For this review, take the finished solid that the model builds, in its own axes (mm). Face numbers are marked on the shaded views. A direction names the side the tool comes from. Give positions to 0.01 mm unless a question says otherwise; leave off trailing zeros. Order: outer loops, then holes, each group sorted by start corner. A loop starts at its lowest first (then second) coordinate and runs counter-clockwise, first axis right, second up.
Item 1: For P1, Ø10, axis at x = 96.5, z = -7.5, coming from the -Y side; P2, Ø4, axis at x = 93, z = -7, coming from the +Y side; P3, Ø10, axis at x = 60.5, y = -6.5, coming from the +Z side, all flat-tipped, find the tip position at first contact; note any pin that passes through.
Item 2: Consider section C-C (x = 74). Give the boundary of the cut face in (y, z).
Item 3: Machinability: for the marked faces 1 and 2, which of the approach directions +Z, -Z, +X, -X, +Y, -Y give a long, thin tool a straight path to every point of the face, cutting with its end or side? Answer none if there is none.
Item 4: Consider section D-D (x = 37.5). Give the boundary of the cut face in (y, z), plus the area to 3 significant figures.
Item 5: For probe 1 along X at (y, z) = (-46, -6); probe 2 along Y at (x, z) = (112, -20.5); probe 3 along Z at (x, y) = (134.5, -69), list the stretches that pass through material, from the lowest coordinate up.
Item 6: Consider section B-B (z = -21.5). Give the boundary of the cut face in (x, y).
Item 7: Consider section A-A (y = -44.45). Give the boundary of the cut face in (x, z) (3 decimals).
Item 8: The part is to be moulded in two halves that separate along Y. For the marked faces 3, 4, 5 and 6, say which applies: released by +Y, released by -Y, zero draft, split by the parting line, or undercut.
```python
from build123d import *

# Parameters (mm, degrees)
F0_W     = 165.1
F0_H     = 31.75
F1_DEPTH = 88.9
F3_DEPTH = 165.101
F4_W     = 165.1
F4_H     = 12.7
F5_DEPTH = 12.7
F6_W     = 165.1
F6_H     = 12.7
F7_DEPTH = 12.7
F8_R     = 12.7
F9_DEPTH = 31.751


with BuildPart() as f1:
    # F0 (on Front) → F1 (new body)
    with BuildSketch(Plane.XZ):
        with Locations((82.55, -15.875)):
            Rectangle(F0_W, F0_H)
    extrude(amount=F1_DEPTH)

    # F2 (on face) → F3 (cut, through all)
    with BuildSketch(Plane.YZ.offset(165.1)):
        Polygon((-70.034593, -19.05), (-69.85, -31.75), (-19.05, -31.75), (-19.05, -19.05), align=None)
    extrude(amount=-F3_DEPTH, mode=Mode.SUBTRACT)

    # F4 (on face) → F5 (cut)
    with BuildSketch(Plane.XZ.offset(88.9)):
        with Locations((82.55, -6.35)):
            Rectangle(F4_W, F4_H)
    extrude(amount=-F5_DEPTH, mode=Mode.SUBTRACT)

    # F6 (on face) → F7 (cut)
    with BuildSketch(Plane(origin=(0, 0, 0), x_dir=(-1, 0, 0), z_dir=(0, 1, 0))):
        with Locations((-82.55, -6.35)):
            Rectangle(F6_W, F6_H)
    extrude(amount=-F7_DEPTH, mode=Mode.SUBTRACT)

    # F8 (on face) → F9 (cut, through all)
    with BuildSketch(Plane.XY):
        with Locations((34.925, -44.45)):
            Circle(F8_R)
        with Locations((130.175, -44.45)):
            Circle(F8_R)
    extrude(amount=-F9_DEPTH, mode=Mode.SUBTRACT)


solid = f1.part
```
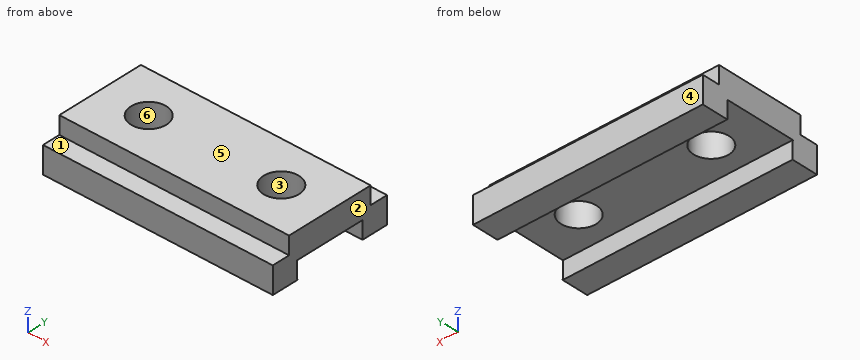
Resolved:
1. P1: stops at y = -76.2
1. P2: stops at y = -12.7
1. P3: stops at z = -12.7
2. outline: (-88.9, -31.75) - (-69.85, -31.75) - (-70.03, -19.05) - (-19.05, -19.05) - (-19.05, -31.75) - (0, -31.75) - (0, -12.7) - (-12.7, -12.7) - (-12.7, 0) - (-76.2, 0) - (-76.2, -12.7) - (-88.9, -12.7) - close
3. face 1: +Z, +X, -X, -Y
3. face 2: +Z, -Z, +X, +Y, -Y
4. outline: (-88.9, -31.75) - (-69.85, -31.75) - (-70.03, -19.05) - (-56.89, -19.05) - (-56.89, 0) - (-76.2, 0) - (-76.2, -12.7) - (-88.9, -12.7) - close; (-32.01, -19.05) - (-19.05, -19.05) - (-19.05, -31.75) - (0, -31.75) - (0, -12.7) - (-12.7, -12.7) - (-12.7, 0) - (-32.01, 0) - close
4. area: 1,380 mm2
5. probe 1: x = 0 to 22.32, 47.53 to 117.57, 142.78 to 165.1
5. probe 2: y = -88.9 to -70.01, -19.05 to 0
5. probe 3: z = -19.05 to 0
6. outline: (0, -88.9) - (165.1, -88.9) - (165.1, -70) - (0, -70) - close; (0, -19.05) - (165.1, -19.05) - (165.1, 0) - (0, 0) - close
7. outline: (0, -19.05) - (22.225, -19.05) - (22.225, 0) - (0, 0) - close; (47.625, -19.05) - (117.475, -19.05) - (117.475, 0) - (47.625, 0) - close; (142.875, -19.05) - (165.1, -19.05) - (165.1, 0) - (142.875, 0) - close
8. face 3: undercut
8. face 4: released by +Y
8. face 5: zero draft
8. face 6: undercut
